```python
from build123d import *

# Parameters (mm, degrees)
ESQUISSE1_W             = 34.5
ESQUISSE1_H             = 32
BOSS_EXTRU_1_DEPTH      = 2
ESQUISSE1_4_W           = 27
ESQUISSE1_4_H           = 29
ESQUISSE1_4_W_2         = 26
ESQUISSE1_4_H_2         = 28
BOSS_EXTRU_2_DEPTH      = 9.5
ESQUISSE6_R             = 3.5
ENL_V_MAT_EXTRU_2_DEPTH = 0.5
ESQUISSE5_R             = 3.5
ENL_V_MAT_EXTRU_3_DEPTH = 0.5


with BuildPart() as part:
    # Esquisse1 → Boss.-Extru.1 (new body)
    with BuildSketch(Plane(origin=(0, 0, 0), x_dir=(1, 0, 0), z_dir=(0, 1, 0))):
        with Locations((-3.171052632, 11.289473684)):
            Rectangle(ESQUISSE1_W, ESQUISSE1_H)
    extrude(amount=BOSS_EXTRU_1_DEPTH)

    # Esquisse1_4 → Boss.-Extru.2 (add)
    with BuildSketch(Plane(origin=(0, 0, 0), x_dir=(1, 0, 0), z_dir=(0, 1, 0))):
        with Locations((-6.921052632, 11.289473684)):
            Rectangle(ESQUISSE1_4_W, ESQUISSE1_4_H)
        with Locations((-6.921052632, 11.289473684)):
            Rectangle(ESQUISSE1_4_W_2, ESQUISSE1_4_H_2, mode=Mode.SUBTRACT)
    extrude(amount=BOSS_EXTRU_2_DEPTH)

    # Esquisse6 → Enl_v. mat.-Extru.2 (cut)
    with BuildSketch(Plane.XY.offset(3.210526316)):
        with Locations((-13.921052632, 9.5)):
            Circle(ESQUISSE6_R)
    extrude(amount=-ENL_V_MAT_EXTRU_2_DEPTH, mode=Mode.SUBTRACT)

    # Esquisse5 → Enl_v. mat.-Extru.3 (cut)
    with BuildSketch(Plane(origin=(0, 0, -25.789473684), x_dir=(-1, 0, 0), z_dir=(0, 0, -1))):
        with Locations((13.921052632, 9.5)):
            Circle(ESQUISSE5_R)
    extrude(amount=-ENL_V_MAT_EXTRU_3_DEPTH, mode=Mode.SUBTRACT)


solid = part.part
```
Work out the finished part from the listing and answer in its coordinate system (mm). A direction names the side the tool comes from. Coordinates: 2 decimals unless noted, no trailing zeros. Loops run counter-clockwise (first coordinate to the right, second up) from the corner with the lowest first, then second, coordinate; pieces in that order, holes last. Notation, with made-up numbers: (81.5, 53.5) - (113.5, 53.5) arc R12 cw to (113.5, 68.5) - close; hole circle Ø10 at (40, 82.5). An arc over 180 degrees is marked (long way). Use a Markdown table: item, result.
Item 1: Consider probe 1 along Z at (x, y) = (-7, 7.5); probe 2 along X at (y, z) = (4.75, -19); probe 3 along Y at (x, z) = (-0.5, -7.5). Determine where each line is inside the solid, lowest interval first. Write a range as from..to.
Evaluation:
| item | result |
|---|---|
| probe 1 | z = -25.79..-25.29, 2.71..3.21 |
| probe 2 | x = -20.42..-19.92, 6.08..6.58 |
| probe 3 | y = 0..2 |
Item 2: For faces 1 (the flat face through (-7, 6, 3.211)), 2 (the flat face through (-7, 6, -25.789)), 3 (the flat face through (-7, 6, 2.711)), determine the directions among +Z, -Z, +X, -X, +Y, -Y from which every point of the face is accessible in a straight line to the end or side of a thin tool.
Evaluation:
| item | result |
|---|---|
| face 1 | +Z, +X, -X, +Y |
| face 2 | -Z, +X, -X, +Y |
| face 3 | +Y |
Item 3: Find section D-D, the plane x = -7. Determine the outline of the cut face in (y, z).
Evaluation:
| item | result |
|---|---|
| outline | (0, -27.29) - (2, -27.29) - (2, -25.79) - (9.5, -25.79) - (9.5, -25.29) - (2, -25.29) - (2, 2.71) - (9.5, 2.71) - (9.5, 3.21) - (2, 3.21) - (2, 4.71) - (0, 4.71) - close |
Item 4: Given pin 1 Ø4 at (x, z) = (-5.5, -17.5) entering from +Y; pin 2 Ø2 at (x, y) = (-8, 6) entering from +Z; pin 3 Ø4 at (y, z) = (7, -9) entering from +X, each flat-ended and moving along its own axis, determine where each tip first touches the part or whether it passes through.
Evaluation:
| item | result |
|---|---|
| pin 1 | stops at y = 2 |
| pin 2 | stops at z = 3.21 |
| pin 3 | stops at x = 6.58 |
Item 5: Find section A-A, the plane y = 8.25. Determine the outline of the cut face in (x, z).
Evaluation:
| item | result |
|---|---|
| outline | (-20.42, -25.79) - (-17.19, -25.79) - (-17.19, -25.29) - (-19.92, -25.29) - (-19.92, 2.71) - (-17.19, 2.71) - (-17.19, 3.21) - (-20.42, 3.21) - close; (-10.65, -25.79) - (6.58, -25.79) - (6.58, 3.21) - (-10.65, 3.21) - (-10.65, 2.71) - (6.08, 2.71) - (6.08, -25.29) - (-10.65, -25.29) - close |
Item 6: Find section B-B, the plane z = -17. Determine the outline of the cut face in (x, y), and give its area (3 significant figures).
Evaluation:
| item | result |
|---|---|
| outline | (-20.42, 0) - (14.08, 0) - (14.08, 2) - (6.58, 2) - (6.58, 9.5) - (6.08, 9.5) - (6.08, 2) - (-19.92, 2) - (-19.92, 9.5) - (-20.42, 9.5) - close |
| area | 76.5 mm2 |
Item 7: The mould has two halves that part along X. Classify faces 4 (the flat face through (-20.26, 9.5, -13.51)), 5 (the flat face through (6.579, 6, -11)), 6 (the cylindrical face through (-13.84, 6, -25.54)): +X half, -X half, draft (parallel to the pull), parting line (faces both ways), or undercut.
Evaluation:
| item | result |
|---|---|
| face 4 | draft |
| face 5 | +X half |
| face 6 | undercut |
Item 8: Find section C-C, the plane y = 3.75. Determine the outline of the cut face in (x, z).
Evaluation:
| item | result |
|---|---|
| outline | (-20.42, -25.79) - (6.58, -25.79) - (6.58, 3.21) - (-20.42, 3.21) - close; hole (-19.92, -25.29) - (6.08, -25.29) - (6.08, 2.71) - (-19.92, 2.71) - close |
